Design review of the part built by this model. Coordinates are the model's own, in mm. Coordinates: 2 decimals unless noted, no trailing zeros. Write each loop counter-clockwise with the first axis right and the second up, starting at its lowest first coordinate (ties: lowest second). Pieces come first, ordered by that corner, then holes. Notation, with made-up numbers: (29.5, -3) -> (37.5, -3) arc R15 cw to (37.5, 6) -> close; hole circle Ø1 at (1.5, -29). An arc over 180 degrees is marked (long way). Write item = value, one per line. Start each with the question number.
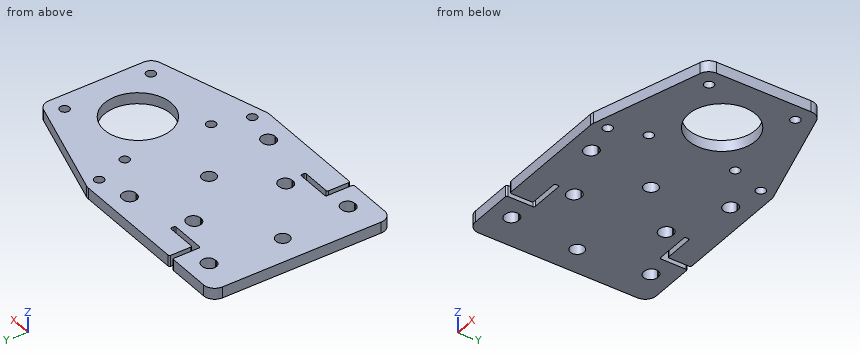
Autodesk Inventor part; units mm, degrees
ref_plane "YZ Plane" through (0, 0, 0) normal (1, 0, 0) x (0, 1, 0)
ref_plane "XZ Plane" through (0, 0, 0) normal (0, 1, 0) x (-1, 0, 0)
ref_plane "XY Plane" through (0, 0, 0) normal (0, 0, 1) x (1, 0, 0)
sketch "Szkic1" plane through (0, 0, 0) normal (0, 0, 1) x (1, 0, 0)
  line L0 (0, 61) -> (0, 4)
  line L1 (106, 15.4829) -> (106, 49.5171)
  line L2 (103.141, 53.3509) -> (64.5584, 64.8338)
  line L3 (103.141, 11.6491) -> (64.5584, 0.1662)
  arc A0 (4, 65) -> (0, 61) centre (4, 61) ccw
  arc A1 (64.5584, 64.8338) -> (63.4174, 65) centre (63.4174, 61) ccw
  arc A2 (106, 49.5171) -> (103.141, 53.3509) centre (102, 49.5171) ccw
  arc A3 (103.141, 11.6491) -> (106, 15.4829) centre (102, 15.4829) ccw
  arc A4 (63.4174, 0) -> (64.5584, 0.1662) centre (63.4174, 4) ccw
  arc A5 (0, 4) -> (4, 0) centre (4, 4) ccw
  line L4 (0, 0) -> (20, 0)
  line L5 (20, 0.5) -> (20, 9.5)
  line L6 (20.5, 10) -> (32.5, 10)
  line L7 (33, 9.5) -> (33, 8.75)
  line L8 (32.5, 8.25) -> (22.25, 8.25)
  line L9 (21.75, 7.75) -> (21.75, 0.5)
  line L10 (4, 0) -> (19.5, 0)
  line L11 (22.25, 0) -> (63.4174, 0)
  arc A6 (19.5, 0) -> (20, 0.5) centre (19.5, 0.5) ccw
  arc A7 (20.5, 10) -> (20, 9.5) centre (20.5, 9.5) ccw
  arc A8 (33, 9.5) -> (32.5, 10) centre (32.5, 9.5) ccw
  arc A9 (32.5, 8.25) -> (33, 8.75) centre (32.5, 8.75) ccw
  arc A10 (22.25, 8.25) -> (21.75, 7.75) centre (22.25, 7.75) ccw
  arc A11 (21.75, 0.5) -> (22.25, 0) centre (22.25, 0.5) ccw
  line L12 (20, 64.5) -> (20, 55.5)
  line L13 (20.5, 55) -> (32.5, 55)
  line L14 (33, 55.5) -> (33, 56.25)
  line L15 (32.5, 56.75) -> (22.25, 56.75)
  line L16 (21.75, 57.25) -> (21.75, 64.5)
  arc A12 (20, 64.5) -> (19.5, 65) centre (19.5, 64.5) ccw
  arc A13 (20, 55.5) -> (20.5, 55) centre (20.5, 55.5) ccw
  arc A14 (32.5, 55) -> (33, 55.5) centre (32.5, 55.5) ccw
  arc A15 (33, 56.25) -> (32.5, 56.75) centre (32.5, 56.25) ccw
  arc A16 (21.75, 57.25) -> (22.25, 56.75) centre (22.25, 57.25) ccw
  arc A17 (22.25, 65) -> (21.75, 64.5) centre (22.25, 64.5) ccw
  line L17 (63.4174, 65) -> (22.25, 65)
  line L18 (19.5, 65) -> (4, 65)
  circle A18 centre (65, 5) radius 1.7
  circle A19 centre (65, 60) radius 1.7
  circle A20 centre (69, 48) radius 1.7
  circle A21 centre (100, 48) radius 1.7
  circle A22 centre (69, 17) radius 1.7
  circle A23 centre (100, 17) radius 1.7
  circle A24 centre (84.5, 32.5) radius 12
  circle A25 centre (9.85, 32.5) radius 2.5
  circle A26 centre (47.85, 32.5) radius 2.5
  arc A27 (11.75, 60) -> (11.75, 55) centre (11.75, 57.5) ccw
  arc A28 (12.25, 55) -> (12.25, 60) centre (12.25, 57.5) ccw
  line L19 (11.75, 60) -> (12.25, 60)
  line L20 (11.75, 55) -> (12.25, 55)
  arc A29 (52.75, 60) -> (52.75, 55) centre (52.75, 57.5) ccw
  arc A30 (53.25, 55) -> (53.25, 60) centre (53.25, 57.5) ccw
  line L21 (52.75, 60) -> (53.25, 60)
  line L22 (52.75, 55) -> (53.25, 55)
  arc A31 (11.75, 10) -> (11.75, 5) centre (11.75, 7.5) ccw
  arc A32 (12.25, 5) -> (12.25, 10) centre (12.25, 7.5) ccw
  line L23 (11.75, 5) -> (12.25, 5)
  line L24 (11.75, 10) -> (12.25, 10)
  arc A33 (52.75, 10) -> (52.75, 5) centre (52.75, 7.5) ccw
  arc A34 (53.25, 5) -> (53.25, 10) centre (53.25, 7.5) ccw
  line L25 (52.75, 5) -> (53.25, 5)
  line L26 (52.75, 10) -> (53.25, 10)
  arc A35 (31.75, 51.5) -> (31.75, 46.5) centre (31.75, 49) ccw
  arc A36 (32.25, 46.5) -> (32.25, 51.5) centre (32.25, 49) ccw
  line L27 (31.75, 51.5) -> (32.25, 51.5)
  line L28 (31.75, 46.5) -> (32.25, 46.5)
  arc A37 (31.75, 18.5) -> (31.75, 13.5) centre (31.75, 16) ccw
  arc A38 (32.25, 13.5) -> (32.25, 18.5) centre (32.25, 16) ccw
  line L29 (31.75, 13.5) -> (32.25, 13.5)
  line L30 (31.75, 18.5) -> (32.25, 18.5)
  point P0 (106, 12.5)
  point P1 (106, 52.5)
  point P2 (20, 10)
  point P3 (33, 10)
  point P4 (33, 8.25)
  point P5 (21.75, 8.25)
  point P6 (21.75, 56.75)
  dimension "d2" = 106
  dimension "d3" = 40
  dimension "d5" = 4
  dimension "d6" = 20
  dimension "d7" = 10
  dimension "d8" = 13
  dimension "d9" = 1.75
  dimension "d10" = 11.25
  dimension "d11" = 0.5
  dimension "d12" = 3.4
  dimension "d13" = 65
  dimension "d14" = 5
  dimension "d16" = 3.4
  dimension "d18" = 69
  dimension "d19" = 3.4
  dimension "d20" = 3.4
  dimension "d21" = 3.4
  dimension "d24" = 69
  dimension "d25" = 31
  dimension "d26" = 31
  dimension "d27" = 24
  dimension "d28" = 84.5
  dimension "d29" = 5
  dimension "d30" = 5
  dimension "d31" = 9.85
  dimension "d32" = 38
  dimension "d33" = 5
  dimension "d35" = 5
  dimension "d36" = 9.25
  dimension "d37" = 5
  dimension "d39" = 5
  dimension "d40" = 35.5
  dimension "d42" = 5
  dimension "d47" = 5
  dimension "d48" = 5
extrude "Płyta1" add sketch "Szkic1" along normal blind 4
equation "\"d49\" = Grubość"
equation "\"PromieńGięcia\" = Grubość"
equation "\"SzerokośćGięciaPodcięcia\" = Grubość"
equation "\"GłębokośćGięciaPodcięcia\" = 0.5 * Grubość"
equation "\"RozmiarPodcięciaNarożnika\" = 4 * Grubość"
equation "\"MinimalnaPozostałość\" = 2 * Grubość"
equation "\"PromieńPrzejścia\" = PromieńGięcia"
equation "\"Rozmiar_promienia_Jacobiego\" = PromieńGięcia"
equation "\"Wielk_odstępu\" = Grubość"
properties part number "podstawa_prawa"
(1) For pin 1 Ø4.5 at (x, y) = (47.85, 32.5) entering from +Z, flat-tipped, find the tip position at first contact; note if it passes through.
(2) Take a section at B-B, the plane y = 23. State the section outline as (x, z) points.
(3) For line 1 (Y direction, x = 100, z = 1.8); line 2 (Y direction, x = 30, z = 1.65); line 3 (Y direction, x = 65.5, z = 3.15), list the stretches that pass through material, from the lowest coordinate up.
(4) Take a section at D-D, the plane z = 2.3. Count the separate pieces of the cut face and the enclosed holes in it, then the cut area to 3 significant figures.
(5) Take a section at C-C, the plane x = 100. State the section outline as (y, z) points, then the cut area to 3 significant figures.
(6) Take a section at A-A, the plane x = 85.5. State the section outline as (y, z) points, then the cut area to 3 significant figures.
Report:
q1.pin_1 = through
q2.outline = (0, 0) -> (77.17, 0) -> (77.17, 4) -> (0, 4) -> close; (91.83, 0) -> (106, 0) -> (106, 4) -> (91.83, 4) -> close
q3.line_1 = 10.71 to 15.3, 18.7 to 46.3, 49.7 to 54.29
q3.line_2 = 0 to 8.25, 10 to 14.21, 17.79 to 47.21, 50.79 to 55, 56.75 to 65
q3.line_3 = 0.45 to 3.38, 6.62 to 58.38, 61.62 to 64.55
q4.separate_pieces = 1
q4.enclosed_holes = 15
q4.area = 5,600 mm2
q5.outline = (10.71, 0) -> (15.3, 0) -> (15.3, 4) -> (10.71, 4) -> close; (18.7, 0) -> (46.3, 0) -> (46.3, 4) -> (18.7, 4) -> close; (49.7, 0) -> (54.29, 0) -> (54.29, 4) -> (49.7, 4) -> close
q5.area = 147 mm2
q6.outline = (6.4, 0) -> (20.54, 0) -> (20.54, 4) -> (6.4, 4) -> close; (44.46, 0) -> (58.6, 0) -> (58.6, 4) -> (44.46, 4) -> close
q6.area = 113 mm2
